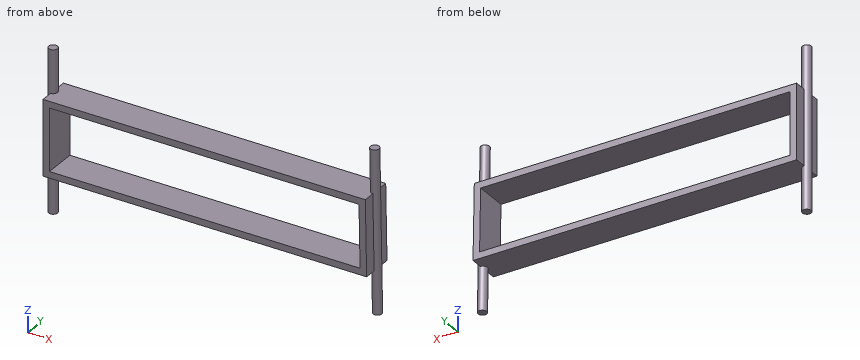
from build123d import *

# Parameters (mm, degrees)
BOSS_EXTRUDE1_DEPTH = 38.1
SKETCH2_R           = 5.08
BOSS_EXTRUDE2_DEPTH = 95.25


with BuildPart() as part:
    # Sketch1 → Boss-Extrude1 (new body)
    with BuildSketch(Plane(origin=(0, 0, 0), x_dir=(1, 0, 0), z_dir=(0, 1, 0))):
        Polygon((-323.509548329, -44.384683315), (57.476455496, -47.650397601), (59.000399511, 41.236539542), (-323.509548329, 44.515316685), align=None)
        Polygon((-315.889548329, -36.829720066), (49.987084067, -39.965920696), (51.24977094, 33.682696008), (-315.889548329, 36.829720066), align=None, mode=Mode.SUBTRACT)
    extrude(amount=-BOSS_EXTRUDE1_DEPTH)

    # Sketch2 → Boss-Extrude2 (add, symmetric)
    with BuildSketch(Plane.XY):
        with Locations((-323.509548329, -19.05)):
            Circle(SKETCH2_R)
    boss_extrude2 = extrude(amount=BOSS_EXTRUDE2_DEPTH, both=True)

    # Mirror1: Boss-Extrude2 across plane
    add(boss_extrude2.mirror(Plane(origin=(-132.612352201, 0, -1.136719062), x_dir=(-0.008571428571427947, 0, 0.9999632646313789), z_dir=(0.999963264631379, 0, 0.008571428571427946))))


solid = part.part
Source: CAD feature listing. Evaluate the final solid. Frame: model axes, mm. Coordinates: 2 decimals unless noted, no trailing zeros. Loops run counter-clockwise (first coordinate to the right, second up) from the corner with the lowest first, then second, coordinate; pieces in that order, holes last. Notation, with made-up numbers: (80, 14) - (134, 14) arc R8 ccw to (134, 18) - close; hole circle Ø6 at (47.5, 0.25). An arc over 180 degrees is marked (long way). One line per question, with ' | ' between items.
1) First-contact query: P1, Ø3, axis at x = -324.5, y = -16.5, coming from the +Z side; P2, Ø5, axis at y = -28.5, z = 48.5, coming from the +X side; P3, Ø7, axis at y = -7.5, z = 4.5, coming from the -X side. Flat tips, straight axial feed; report the tip coordinate or a pass-through.
Report:
P1: stops at z = 95.25 | P2: stops at x = 57.5 | P3: stops at x = -323.51
2) Section A-A, the plane y = -8.5. Return loops of the section in (x, z), then the cut area to 3 significant figures.
Report:
outline: (-323.51, -44.52) - (59, -41.24) - (57.48, 47.65) - (-323.51, 44.38) - close; hole (-315.89, -36.83) - (51.25, -33.68) - (49.99, 39.97) - (-315.89, 36.83) - close | area: 6,940 mm²
3) Line query: line 1 along Z through (x, y) = (-287.5, -11.5); line 2 along Z through (x, y) = (-147.5, -26); line 3 along X through (y, z) = (-19, -77). Output: solid intervals per line, ascending.
Report:
line 1: z = -44.21 to -36.59, 37.07 to 44.69 | line 2: z = -43.01 to -35.39, 38.27 to 45.89 | line 3: x = -328.59 to -318.43, 54.53 to 64.69
4) Section B-B, the plane x = -278. Return loops of the section in (y, z), then the cut area to 3 significant figures.
Report:
outline: (-38.1, -44.13) - (0, -44.13) - (0, -36.5) - (-38.1, -36.5) - close; (-38.1, 37.15) - (0, 37.15) - (0, 44.77) - (-38.1, 44.77) - close | area: 581 mm²
